Autodesk Inventor part; units mm, degrees
ref_plane "YZ Plane" through (0, 0, 0) normal (1, 0, 0) x (0, 1, 0)
ref_plane "XZ Plane" through (0, 0, 0) normal (0, 1, 0) x (-1, 0, 0)
ref_plane "XY Plane" through (0, 0, 0) normal (0, 0, 1) x (1, 0, 0)
sketch "Sketch1" plane through (0, 0, 0) normal (0, 0, 1) x (1, 0, 0)
  line L0 (-32.5, -42.5) -> (32.5, -42.5)
  line L1 (32.5, -42.5) -> (32.5, 42.5)
  line L2 (32.5, 42.5) -> (-32.5, 42.5)
  line L3 (-32.5, 42.5) -> (-32.5, -42.5)
  line L4 (-32.5, -42.5) -> (32.5, 42.5) construction
  line L5 (32.5, -42.5) -> (-32.5, 42.5) construction
  line L6 (15.25, -15.25) -> (-15.25, -15.25)
  line L7 (-15.25, -15.25) -> (-15.25, 15.25)
  line L8 (-15.25, 15.25) -> (15.25, 15.25)
  line L9 (15.25, 15.25) -> (15.25, -15.25)
  line L10 (15.25, -15.25) -> (-15.25, 15.25) construction
  line L11 (-15.25, -15.25) -> (15.25, 15.25) construction
  point P0 (0, 0)
  dimension "d154" = 65
  dimension "d155" = 85
  dimension "d172" = 30.5
extrude "Plate5" add sketch "Sketch1" along normal blind 3
sketch "Sketch9" plane through (0, 0, 3) normal (0, 0, 1) x (1, 0, 0)
  circle A0 centre (25, -35) radius 4.5
  line L0 (25, 35) -> (-25, 35) construction
  line L1 (-25, 35) -> (-25, -35) construction
  line L2 (-25, -35) -> (25, -35) construction
  line L3 (25, -35) -> (25, 35) construction
  line L4 (25, 35) -> (-25, -35) construction
  line L5 (-25, 35) -> (25, -35) construction
  circle A1 centre (-25, -35) radius 4.5
  circle A2 centre (25, 35) radius 4.5
  circle A3 centre (-25, 35) radius 4.5
  point P0 (0, 0)
  dimension "d173" = 70
  dimension "d174" = 9
  dimension "d175" = 50
extrude "Cut2" cut sketch "Sketch9" against normal blind 3
fillet "Corner Round1" radius 6 4 edges at (32.5, 42.5, 1.5) (-32.5, 42.5, 1.5) (-32.5, -42.5, 1.5) (32.5, -42.5, 1.5)
fillet "Corner Round2" radius 1 4 edges at (-15.25, 15.25, 1.5) (-15.25, -15.25, 1.5) (15.25, -15.25, 1.5) (15.25, 15.25, 1.5)
properties part number "APN 760 FDS 1200 FLANGE 3" material "Stainless Steel"
Geometry check sheet. Reference: the model listing, model coordinates, mm. A direction names the side the tool comes from. Coordinates: 2 decimals unless noted, no trailing zeros. Order: outer loops, then holes, each group sorted by start corner. A loop starts at its lowest first (then second) coordinate and runs counter-clockwise, first axis right, second up. Notation, with made-up numbers: (83.25, -1.75) - (93.25, -1.75) arc R10 cw to (93.25, 8.25) - close; hole circle Ø5 at (83, -32). An arc over 180 degrees is marked (long way). Answer as a JSON object with one key per item and string values. Group by question number.
Item 1: Sectioned sample at B-B, the plane y = 35. Record the cut outline in (x, z), and give its area (3 significant figures).
Item 2: Sectioned sample at A-A, the plane x = -25. Record the cut outline in (y, z), and give its area (3 significant figures).
Item 3: Tool access check on faces 5 (the face through (0, 19, 3)), 6 (the face through (15.25, 0, 1)). Record the directions out of +Z, -Z, +X, -X, +Y, -Y that give a thin tool (end or side, any length) a straight path to the whole face; none if there is none.
Item 4: Scan lines: probe 1 along Y at (x, z) = (25, 1.75); probe 2 along Y at (x, z) = (9.5, 1.5); probe 3 along X at (y, z) = (-9.5, 2). Record each from-to range of solid material in increasing order.
Item 5: Sectioned sample at D-D, the plane y = 5. Record the cut outline in (x, z), and give its area (4 significant figures).
Item 6: Sectioned sample at C-C, the plane z = 0.7. Record the cut outline in (x, y), and give its area (3 significant figures).
Item 7: Draft check along X on faces 1 (the face through (24.02, -39.39, 1.52)), 2 (the face through (0, 19, 0)), 3 (the face through (-30.789, -40.696, 1.521)), 4 (the face through (30.789, 40.696, 1.521)). Enter one of: +X half, -X half, draft (parallel to the pull), parting line (faces both ways), or undercut.
Resolved:
{
 "1": {"outline": "(-32.5, 0) - (-29.5, 0) - (-29.5, 3) - (-32.5, 3) - close; (-20.5, 0) - (20.5, 0) - (20.5, 3) - (-20.5, 3) - close; (29.5, 0) - (32.5, 0) - (32.5, 3) - (29.5, 3) - close", "area": "141 mm^2"},
 "2": {"outline": "(-42.5, 0) - (-39.5, 0) - (-39.5, 3) - (-42.5, 3) - close; (-30.5, 0) - (30.5, 0) - (30.5, 3) - (-30.5, 3) - close; (39.5, 0) - (42.5, 0) - (42.5, 3) - (39.5, 3) - close", "area": "201 mm^2"},
 "3": {"face 5": "+Z, +X, -X, +Y, -Y", "face 6": "+Z, -Z"},
 "4": {"probe 1": "-42.5 to -39.5, -30.5 to 30.5, 39.5 to 42.5", "probe 2": "-42.5 to -15.25, 15.25 to 42.5", "probe 3": "-32.5 to -15.25, 15.25 to 32.5"},
 "5": {"outline": "(-32.5, 0) - (-15.25, 0) - (-15.25, 3) - (-32.5, 3) - close; (15.25, 0) - (32.5, 0) - (32.5, 3) - (15.25, 3) - close", "area": "103.5 mm^2"},
 "6": {"outline": "(-32.5, -36.5) arc R6 ccw to (-26.5, -42.5) - (26.5, -42.5) arc R6 ccw to (32.5, -36.5) - (32.5, 36.5) arc R6 ccw to (26.5, 42.5) - (-26.5, 42.5) arc R6 ccw to (-32.5, 36.5) - close; hole circle Ø9 at (-25, -35); hole circle Ø9 at (-25, 35); hole (-15.25, -14.25) arc R1 ccw to (-14.25, -15.25) - (14.25, -15.25) arc R1 ccw to (15.25, -14.25) - (15.25, 14.25) arc R1 ccw to (14.25, 15.25) - (-14.25, 15.25) arc R1 ccw to (-15.25, 14.25) - close; hole circle Ø9 at (25, -35); hole circle Ø9 at (25, 35)", "area": "4,310 mm^2"},
 "7": {"face 1": "undercut", "face 2": "draft", "face 3": "-X half", "face 4": "+X half"}
}
